The figure shows three views and two pictorial views of one solid part (mm, origin at its lowest corner). Answer the questions. A direction names the side the tool comes from. Coordinates: 2 decimals unless noted, no trailing zeros. Order: outer loops, then holes, each group sorted by start corner. A loop starts at its lowest first (then second) coordinate and runs counter-clockwise, first axis right, second up. Notation, with made-up numbers: (65.5, 52.5) -> (85.5, 52.5) arc R26 cw to (85.5, 82.5) -> close; hole circle Ø1 at (80.25, -0.5). An arc over 180 degrees is marked (long way). Write item = value, one per line. Start each with the question number.
Q1. Straight lines are drawn through the part: L1, parallel to Y at x = 1.25, z = 5.75 (1 decimal); L2, parallel to Y at x = 0.75, z = 4.5 (1 decimal); L3, parallel to Z at x = 7.5, y = 11.25 (1 decimal). For each, find the intervals that lie inside material, in ascending order. Write a range as from..to.
Q2. Which of the six approach directions +Z, -Z, +X, -X, +Y, -Y give full straight-line access (tool end or side, diameter ignored) to the marked faces 1, 2 and 3?
Q3. The part is cut by section A-A, the plane y = 15. Determine the outline of the cut face in (x, z).
Q4. The part is cut by section D-D, the plane y = 26.25. Determine the outline of the cut face in (x, z), plus the area to 3 significant figures.
Q5. Flat-ended cylindrical pins translate along their axes: pin 1 (2 mm diameter, centred on x = 5.5, z = 1.5, fed in from +Y); pin 2 (1 mm diameter, centred on x = 3.5, y = 4, fed in from -Z) (1 decimal); pin 3 (1.5 mm diameter, centred on x = 1, z = 9.5, fed in from +Y); pin 4 (1.9 mm diameter, centred on y = 4.5, z = 6, fed in from -X). Find the tip coordinate at first contact, or state that the pin passes through.
Q6. For a pull along Y with two mould halves and no side action, classify the marked faces 4, 5 and 6 as +Y half, -Y half, draft (parallel to the pull), parting line (faces both ways), or undercut.
Q7. The part is cut by section C-C, the plane z = 9.5. Determine the outline of the cut face in (x, y), plus the area to 3 significant figures.
Q8. The part is cut by section B-B, the plane x = 2.5. Count the separate pieces of the cut face and the enclosed holes in it, plus the area to 3 significant figures.
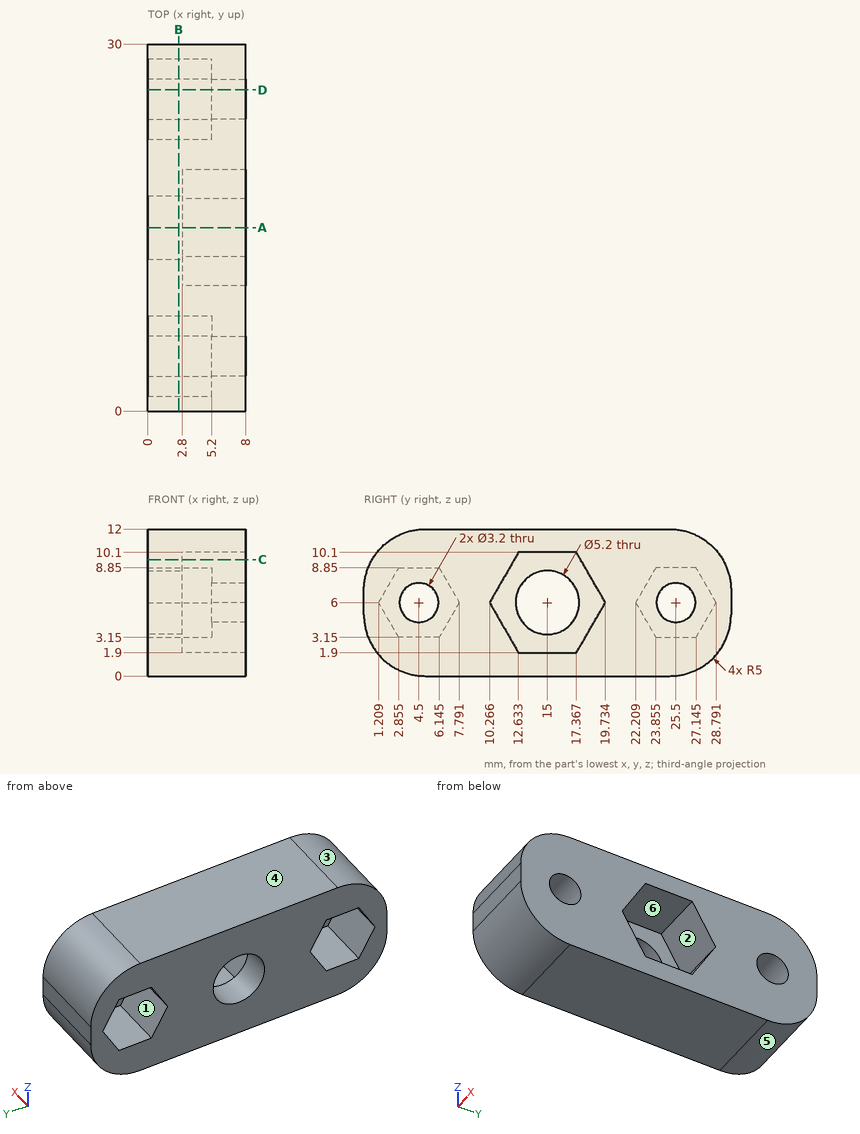
Model answer:
q1.L1 = 0..1.4, 7.6..12.4, 17.6..22.4, 28.6..30
q1.L2 = 0..2.1, 6.9..12.9, 17.1..23.1, 27.9..30
q1.L3 = 0..4.3, 7.7..12
q2.face_1 = -X
q2.face_2 = +X
q2.face_3 = +Z, +X, -X, -Y
q3.outline = (0, 0) -> (8, 0) -> (8, 1.9) -> (2.8, 1.9) -> (2.8, 3.4) -> (0, 3.4) -> close; (0, 8.6) -> (2.8, 8.6) -> (2.8, 10.1) -> (8, 10.1) -> (8, 12) -> (0, 12) -> close
q4.outline = (0, 0.16) -> (8, 0.16) -> (8, 4.59) -> (5.2, 4.59) -> (5.2, 3.15) -> (0, 3.15) -> close; (0, 8.85) -> (5.2, 8.85) -> (5.2, 7.41) -> (8, 7.41) -> (8, 11.84) -> (0, 11.84) -> close
q4.area = 55.9 mm2
q5.pin_1 = 29.33
q5.pin_2 = 0
q5.pin_3 = 29.68
q5.pin_4 = through
q6.face_4 = draft
q6.face_5 = +Y half
q6.face_6 = undercut
q7.outline = (0, 0.67) -> (8, 0.67) -> (8, 12.29) -> (2.8, 12.29) -> (2.8, 17.71) -> (8, 17.71) -> (8, 29.33) -> (0, 29.33) -> close
q7.area = 201 mm2
q8.separate_pieces = 1
q8.enclosed_holes = 3
q8.area = 261 mm2
